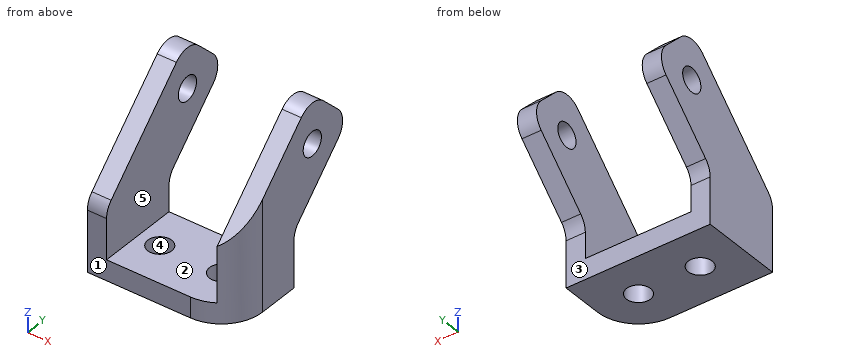
```python
from build123d import *

# Parameters (mm, degrees)
F0_W        = 21
F0_H        = 12
F0_R        = 1.75
F1_DEPTH    = 3
F3_R        = 1.75
F4_DEPTH    = 2.8
F2_R        = 1.75
F5_DEPTH    = 2.8
F6_R        = 6
F7_T1_DEPTH = 2.8
F7_T3_DEPTH = 2.8
F7_T5_DEPTH = 17.8
F7_T7_DEPTH = 17.8
F7_T9_DEPTH = 9.0132034356


# Not quite as in the source:
# - a fillet or chamfer that OpenCascade refuses, or shapes differently, is made with other operations: its cross-section is extruded or revolved along the edge and cut away or added


with BuildPart() as f1:
    # F0 (on Top) → F1 (new body)
    with BuildSketch(Plane.XY):
        with Locations((10.5, 6)):
            Rectangle(F0_W, F0_H)
        with Locations((6, 6)):
            Circle(F0_R, mode=Mode.SUBTRACT)
        with Locations((15, 6)):
            Circle(F0_R, mode=Mode.SUBTRACT)
    extrude(amount=F1_DEPTH)

    # F3 (on face) → F4 (join)
    with BuildSketch(Plane.YZ.offset(21)):
        Polygon((0, 10.1421356237), (0, 3), (12, 3), (12, 8), (22.6066017178, 18.6066017178), (15.5355339059, 25.6776695297), align=None)
        with Locations((15.5355339059, 18.6066017178)):
            Circle(F3_R, mode=Mode.SUBTRACT)
    extrude(amount=-F4_DEPTH)

    # F2 (on face) → F5 (join)
    with BuildSketch(Plane(origin=(0, 0, 0), x_dir=(0, -1, 0), z_dir=(-1, 0, 0))):
        Polygon((-12, 8), (-12, 3), (0, 3), (0, 10.1421356237), (-15.5355339059, 25.6776695297), (-22.6066017178, 18.6066017178), align=None)
        with Locations((-15.5355339059, 18.6066017178)):
            Circle(F2_R, mode=Mode.SUBTRACT)
    extrude(amount=-F5_DEPTH)

    # F6
    f6_edges = [f1.edges().sort_by_distance(p)[0] for p in [
        (21, 0, 5.071068),
    ]]
    fillet(f6_edges, radius=F6_R)

    # F7: fillet of radius 3 on 8 edges, made by hand

    # F7_s2 → F7_t1 (join)
    with BuildSketch(Plane.YZ.offset(18.2)):
        with BuildLine():
            ThreePointArc((12, 6.7573593129), (12.2283614025, 7.90540961), (12.8786796564, 8.8786796564))
            Line((12.8786796564, 8.8786796564), (12, 8))
            Line((12, 8), (12, 6.7573593129))
        make_face()
    extrude(amount=F7_T1_DEPTH)

    # F7_s4 → F7_t3 (join)
    with BuildSketch(Plane.YZ):
        with BuildLine():
            ThreePointArc((12, 6.7573593129), (12.2283614025, 7.90540961), (12.8786796564, 8.8786796564))
            Line((12.8786796564, 8.8786796564), (12, 8))
            Line((12, 8), (12, 6.7573593129))
        make_face()
    extrude(amount=F7_T3_DEPTH)

    # F7_s6 → F7_t5 (cut)
    with BuildSketch(Plane.YZ.offset(-7.5)):
        with BuildLine():
            ThreePointArc((20.4852813742, 20.7279220614), (21.3639610307, 18.6066017178), (20.4852813742, 16.4852813742))
            Line((20.4852813742, 16.4852813742), (22.6066017178, 18.6066017178))
            Line((22.6066017178, 18.6066017178), (20.4852813742, 20.7279220614))
        make_face()
        with BuildLine():
            ThreePointArc((13.4142135624, 23.5563491861), (15.5355339059, 24.4350288425), (17.6568542495, 23.5563491861))
            Line((17.6568542495, 23.5563491861), (15.5355339059, 25.6776695297))
            Line((15.5355339059, 25.6776695297), (13.4142135624, 23.5563491861))
        make_face()
    extrude(amount=F7_T5_DEPTH, mode=Mode.SUBTRACT)

    # F7_s8 → F7_t7 (cut)
    with BuildSketch(Plane.YZ.offset(10.7)):
        with BuildLine():
            ThreePointArc((20.4852813742, 20.7279220614), (21.3639610307, 18.6066017178), (20.4852813742, 16.4852813742))
            Line((20.4852813742, 16.4852813742), (22.6066017178, 18.6066017178))
            Line((22.6066017178, 18.6066017178), (20.4852813742, 20.7279220614))
        make_face()
        with BuildLine():
            ThreePointArc((13.4142135624, 23.5563491861), (15.5355339059, 24.4350288425), (17.6568542495, 23.5563491861))
            Line((17.6568542495, 23.5563491861), (15.5355339059, 25.6776695297))
            Line((15.5355339059, 25.6776695297), (13.4142135624, 23.5563491861))
        make_face()
    extrude(amount=F7_T7_DEPTH, mode=Mode.SUBTRACT)

    # F7_s10 → F7_t9 (cut)
    with BuildSketch(Plane.YZ.offset(-3.1066017178)):
        with BuildLine():
            ThreePointArc((0, 8.8994949366), (0.2283614025, 10.0475452337), (0.8786796564, 11.0208152802))
            Line((0.8786796564, 11.0208152802), (0, 10.1421356237))
            Line((0, 10.1421356237), (0, 8.8994949366))
        make_face()
    extrude(amount=F7_T9_DEPTH, mode=Mode.SUBTRACT)


solid = f1.part
```
For this review, take the finished solid that the model builds, in its own axes (mm). Face numbers are marked on the shaded views. A direction names the side the tool comes from. Give positions to 0.01 mm unless a question says otherwise; leave off trailing zeros. Loops run counter-clockwise (first coordinate to the right, second up) from the corner with the lowest first, then second, coordinate; pieces in that order, holes last. Notation, with made-up numbers: M 70.5,62.25 L 128.5,62.25 A12 cw 128.5,67.25 Z; hole C 87.5,61 d9. An arc over 180 degrees is marked long. One line per item, written item: value. Start each with the question number.
Q1. Machinability: for the marked faces 1 and 2, which of the approach directions +Z, -Z, +X, -X, +Y, -Y give a long, thin tool a straight path to every point of the face, cutting with its end or side? Answer none if there is none.
Q2. Add section C-C (z = 11.75). Give the boundary of the cut face in (x, y).
Q3. For L1, parallel to X at y = 9.25, z = 3.5; L2, parallel to Z at x = 15, y = 9; L3, parallel to X at y = 3.25, z = 12.5, list the stretches that pass through material, from the lowest coordinate up.
Q4. Add section D-D (y = 5). Give the boundary of the cut face in (x, z), and give its area (3 significant figures).
Q5. Add section B-B (y = 18.5). Give the boundary of the cut face in (x, z), and give its area (3 significant figures).
Q6. Add section A-A (x = 6). Give the boundary of the cut face in (y, z).
Q7. Draft analysis for pull direction Y (two halves, no side actions). For the marked faces 3, 4 and 5, state which applies: released by +Y, released by -Y, zero draft, split by the parting line, or undercut.
Q8. Clearance check with flat-ended pins moving along their axes: pin 1 Ø3 at (x, y) = (15, 6) entering from -Z; pin 2 Ø7.5 at (x, z) = (11, 4.5) entering from +Y; pin 3 Ø4.5 at (x, y) = (6, 6) entering from +Z; pin 4 Ø10 at (x, y) = (3.5, 4.5) entering from +Z. State where each tip first meets the part, or that it passes through.
Reply:
1. face 1: +Z, -Z, +X, -X, -Y
1. face 2: +Z, +Y, -Y
2. outline: M 0,1.61 L 2.8,1.61 L 2.8,15.75 L 0,15.75 Z; M 18.2,1.61 L 19.09,1.61 A6 ccw 21,6 L 21,15.75 L 18.2,15.75 Z
3. L1: 0 to 2.8, 18.2 to 21
3. L2: 0 to 3
3. L3: 0 to 2.8, 18.2 to 20.33
4. outline: M 0,0 L 4.56,0 L 4.56,3 L 2.8,3 L 2.8,15.14 L 0,15.14 Z; M 7.44,0 L 13.56,0 L 13.56,3 L 7.44,3 Z; M 16.44,0 L 20.92,0 L 20.92,15.14 L 18.2,15.14 L 18.2,3 L 16.44,3 Z
4. area: 112 mm²
5. outline: M 0,14.5 L 2.8,14.5 L 2.8,22.71 L 0,22.71 Z; M 18.2,14.5 L 21,14.5 L 21,22.71 L 18.2,22.71 Z
5. area: 46.0 mm²
6. outline: M 0,0 L 4.25,0 L 4.25,3 L 0,3 Z; M 7.75,0 L 12,0 L 12,3 L 7.75,3 Z
7. face 3: released by +Y
7. face 4: undercut
7. face 5: zero draft
8. pin 1: through
8. pin 2: y = 12
8. pin 3: z = 3
8. pin 4: z = 19.59
